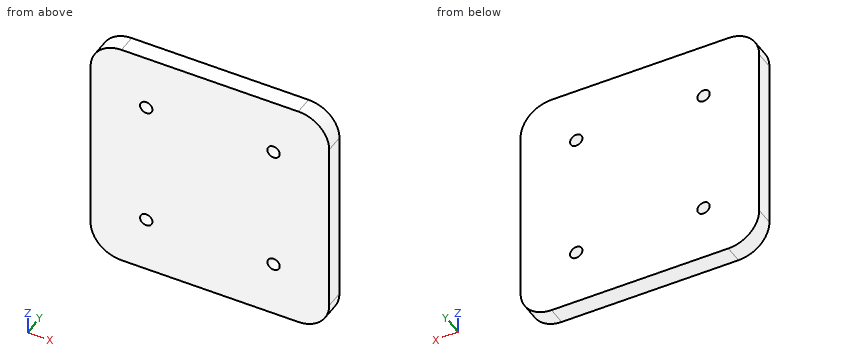
```python
from build123d import *

# Parameters (mm, degrees)
CROQUIS1_W              = 77.15
CROQUIS1_H              = 77.15
SALIENTE_EXTRUIR1_DEPTH = 6
CROQUIS2_R              = 2
CORTAR_EXTRUIR1_DEPTH   = 40
REDONDEO1_R             = 10


with BuildPart() as part:
    # Croquis1 → Saliente-Extruir1 (new body)
    with BuildSketch(Plane.XZ.offset(-65.5)):
        with Locations((63.993998695, -38.595)):
            Rectangle(CROQUIS1_W, CROQUIS1_H)
    extrude(amount=-SALIENTE_EXTRUIR1_DEPTH)

    # Croquis2 → Cortar-Extruir1 (cut)
    with BuildSketch(Plane(origin=(0, 71.5, 0), x_dir=(1, 0, 0), z_dir=(0, 1, 0))):
        with Locations((84.568998695, 59.17)):
            Circle(CROQUIS2_R)
        with Locations((84.568998695, 18.02)):
            Circle(CROQUIS2_R)
        with Locations((43.418998695, 18.02)):
            Circle(CROQUIS2_R)
        with Locations((43.418998695, 59.17)):
            Circle(CROQUIS2_R)
    extrude(amount=-CORTAR_EXTRUIR1_DEPTH, mode=Mode.SUBTRACT)

    # Redondeo1
    redondeo1_edges = [part.edges().sort_by_distance(p)[0] for p in [
        (25.418998695, 68.5, -0.02),
        (102.568998695, 68.5, -0.02),
        (102.568998695, 68.5, -77.17),
        (25.418998695, 68.5, -77.17),
    ]]
    fillet(redondeo1_edges, radius=REDONDEO1_R)


solid = part.part
```
Part model, mm, in its own coordinate system. Give positions to 0.01 mm unless a question says otherwise; leave off trailing zeros. Order: outer loops, then holes, each group sorted by start corner. A loop starts at its lowest first (then second) coordinate and runs counter-clockwise, first axis right, second up. Notation, with made-up numbers: M -0.75,74.5 L 43.25,74.5 A26 cw 43.25,105.5 Z; hole C 15,15 d11. An arc over 180 degrees is marked long. Use a Markdown table: item, result. Add a question column.
(1) Saw through at B-B, the plane z = -18.02. Give the cut face in (x, y), and give its area (3 significant figures).
(2) Saw through at A-A, the plane y = 68.25. Give the cut face in (x, z), and give its area (3 significant figures).
(3) Saw through at C-C, the plane x = 85. Give the cut face in (y, z).
(4) Drop a flat-ended pin along its axis: P1, Ø6.5, axis at x = 43.42, z = -18.02, coming from the +Y side. Give the stop position or say it passes through.
(5) Probe line 1 along X through (y, z) = (68.1, -18.02); line 2 along Z through (x, y) = (94.5, 66); line 3 along X through (y, z) = (67.8, -73.5). List the from-to ranges inside material, lowest first. Write a range as [from, to].
Answer key:
| question | item | result |
|---|---|---|
| 1 | outline | M 25.42,65.5 L 41.42,65.5 L 41.42,71.5 L 25.42,71.5 Z; M 45.42,65.5 L 82.57,65.5 L 82.57,71.5 L 45.42,71.5 Z; M 86.57,65.5 L 102.57,65.5 L 102.57,71.5 L 86.57,71.5 Z |
| 1 | area | 415 mm^2 |
| 2 | outline | M 25.42,-67.17 A10 ccw 35.42,-77.17 L 92.57,-77.17 A10 ccw 102.57,-67.17 L 102.57,-10.02 A10 ccw 92.57,-0.02 L 35.42,-0.02 A10 ccw 25.42,-10.02 Z; hole C 43.42,-59.17 d4; hole C 43.42,-18.02 d4; hole C 84.57,-59.17 d4; hole C 84.57,-18.02 d4 |
| 2 | area | 5,820 mm^2 |
| 3 | outline | M 65.5,-77.17 L 71.5,-77.17 L 71.5,-61.12 L 65.5,-61.12 Z; M 65.5,-57.22 L 71.5,-57.22 L 71.5,-19.97 L 65.5,-19.97 Z; M 65.5,-16.07 L 71.5,-16.07 L 71.5,-0.02 L 65.5,-0.02 Z |
| 4 | P1 | y = 71.5 |
| 5 | line 1 | [25.42, 41.42], [45.42, 82.57], [86.57, 102.57] |
| 5 | line 2 | [-76.98, -0.21] |
| 5 | line 3 | [27.68, 100.31] |
